Part model, mm, in its own coordinate system. Give positions to 0.01 mm unless a question says otherwise; leave off trailing zeros. Write each loop counter-clockwise with the first axis right and the second up, starting at its lowest first coordinate (ties: lowest second). Pieces come first, ordered by that corner, then holes. Notation, with made-up numbers: (-19, 70) - (38, 70) arc R19 ccw to (38, 95) - close; hole circle Ø11 at (44.25, 27.25). An arc over 180 degrees is marked (long way). Answer in a Markdown table with one row per item. Add a question column.
1. Drop flat-ended pins along their axis: pin 1 Ø6 at (x, y) = (10.5, 102.5) entering from -Z; pin 2 Ø3.5 at (x, y) = (10, 12) entering from +Z; pin 3 Ø1 at (y, z) = (173, -10.5) entering from -X; pin 4 Ø4 at (y, z) = (51, -10) entering from -X. Give the stop position or say it passes through.
2. Probe line 1 along Y through (x, z) = (10, -13.75); line 2 along X through (y, z) = (39, -10); line 3 along X through (y, z) = (70, -5.5). List the from-to ranges inside material, lowest first.
3. Pull direction X, two halves, no side cores. Call faces 1 (the flat face through (3, 148, 0)), 2 (the cylindrical face through (12.77, 41.41, -8.85)), 3 (the flat face through (0, 148, -16)): released by +X, released by -X, zero draft, split by the parting line, or undercut.
4. Band-saw the part on A-A on y = 266.5. Write the cut outline in (x, z), plus the area to 3 significant figures.
```python
from build123d import *

# Parameters (mm, degrees)
SKIZZE1_W                       = 20
SKIZZE1_H                       = 20
AUFSATZ_LINEAR_AUSTRAGEN1_DEPTH = 300
SCHNITT_LINEAR_AUSTRAGEN1_DEPTH = 301
SKIZZE3_R                       = 3
SCHNITT_LINEAR_AUSTRAGEN2_DEPTH = 301
SKETCH1_R                       = 3
CUT_EXTRUDE1_DEPTH              = 21


with BuildPart() as part:
    # Skizze1 → Aufsatz-Linear austragen1 (new body)
    with BuildSketch(Plane(origin=(0, 0, 0), x_dir=(1, 0, 0), z_dir=(0, 1, 0))):
        with Locations((10, 10)):
            Rectangle(SKIZZE1_W, SKIZZE1_H)
    extrude(amount=AUFSATZ_LINEAR_AUSTRAGEN1_DEPTH)

    # Skizze2 → Schnitt-Linear austragen1 (cut, through all)
    with BuildSketch(Plane(origin=(0, 300, 0), x_dir=(1, 0, 0), z_dir=(0, 1, 0))):
        Polygon((7, 20), (10, 17), (13, 20), align=None)
        Polygon((20, 13), (17, 10), (20, 7), align=None)
        Polygon((0, 7), (0, 13), (3, 10), align=None)
        Polygon((7, 0), (13, 0), (10, 3), align=None)
    extrude(amount=-SCHNITT_LINEAR_AUSTRAGEN1_DEPTH, mode=Mode.SUBTRACT)

    # Skizze3 → Schnitt-Linear austragen2 (cut, through all)
    with BuildSketch(Plane(origin=(0, 300, 0), x_dir=(1, 0, 0), z_dir=(0, 1, 0))):
        with Locations((10, 10)):
            Circle(SKIZZE3_R)
    extrude(amount=-SCHNITT_LINEAR_AUSTRAGEN2_DEPTH, mode=Mode.SUBTRACT)

    # Sketch1 → Cut-Extrude1 (cut, through all)
    with BuildSketch(Plane.XY):
        with Locations((10, 12)):
            Circle(SKETCH1_R)
        with Locations((10, 70)):
            Circle(SKETCH1_R)
    extrude(amount=-CUT_EXTRUDE1_DEPTH, mode=Mode.SUBTRACT)


solid = part.part
```
Values:
| question | item | result |
|---|---|---|
| 1 | pin 1 | stops at z = -20 |
| 1 | pin 2 | passes through |
| 1 | pin 3 | stops at x = 2 |
| 1 | pin 4 | stops at x = 1 |
| 2 | line 1 | y = 0 to 9, 15 to 67, 73 to 300 |
| 2 | line 2 | x = 3 to 7, 13 to 17 |
| 2 | line 3 | x = 0 to 7, 13 to 20 |
| 3 | face 1 | zero draft |
| 3 | face 2 | undercut |
| 3 | face 3 | released by -X |
| 4 | outline | (0, -20) - (7, -20) - (10, -17) - (13, -20) - (20, -20) - (20, -13) - (17, -10) - (20, -7) - (20, 0) - (13, 0) - (10, -3) - (7, 0) - (0, 0) - (0, -7) - (3, -10) - (0, -13) - close; hole circle Ø6 at (10, -10) |
| 4 | area | 336 mm² |
